Job drawing, mm, ordinate dimensions from the low corner. One solid piece. Give positions to 0.01 mm unless a question says otherwise; leave off trailing zeros. Write each loop counter-clockwise with the first axis right and the second up, starting at its lowest first coordinate (ties: lowest second). Pieces come first, ordered by that corner, then holes. Notation, with made-up numbers: (-6.5, -19) - (0.5, -19) arc R25 ccw to (0.5, 14) - close; hole circle Ø8 at (14.25, -17). An arc over 180 degrees is marked (long way). Answer as a JSON object with one key per item and string values.
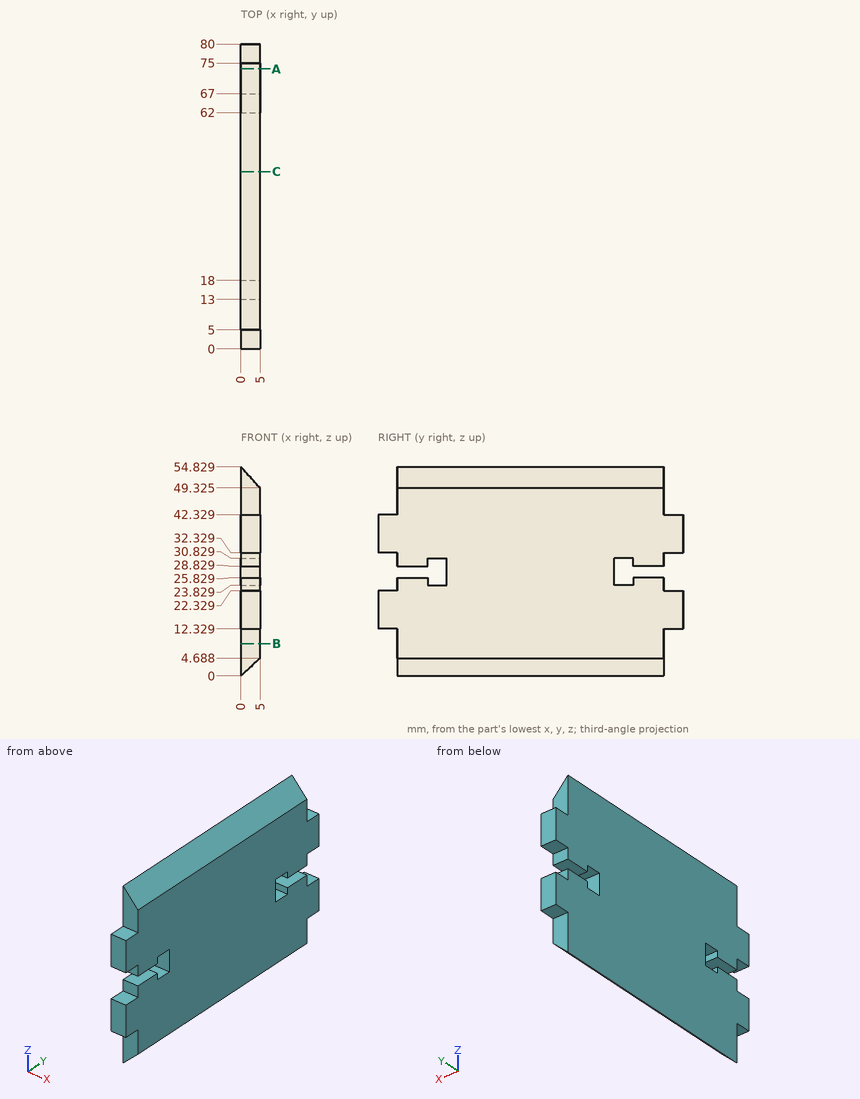
Item 1: Cut at C-C (y = 46.5). Give the cut face in (x, z) (3 decimals), and give its area (3 significant figures).
Entries:
{"outline": "(0, 0) - (5, 4.688) - (5, 49.325) - (0, 54.829) - close", "area": "249 mm2"}
Item 2: Flat gauge pins, fed straight in: P1, Ø1.5, axis at x = 3.5, z = 4.5, coming from the -Y side; P2, Ø2.5, axis at x = 3, y = 63.5, coming from the +Z side; P3, Ø1.5, axis at x = 3.5, y = 70.5, coming from the +Z side. Where does each tip first touch, or does it go through?
Entries:
{"P1": "y = 5", "P2": "z = 52.9", "P3": "z = 51.8"}
Item 3: Cut at B-B (z = 8.5). Give the cut face in (x, y).
Entries:
{"outline": "(0, 5) - (5, 5) - (5, 75) - (0, 75) - close"}
Item 4: Probe line 1 (Y direction, x = 1.9, z = 24.5); line 2 (Y direction, x = 4.25, z = 22.5); line 3 (Z direction, x = 2.95, y = 17.5). List the from-to ranges inside material, lowest first. Write a range as from..to.
Entries:
{"line 1": "5..13, 18..62, 67..75", "line 2": "5..75", "line 3": "2.77..23.83, 30.83..51.58"}
Item 5: Cut at A-A (y = 73.5). Give the cut face in (x, z) (3 decimals), and give its area (3 significant figures).
Entries:
{"outline": "(0, 0) - (5, 4.688) - (5, 25.829) - (0, 25.829) - close; (0, 28.829) - (5, 28.829) - (5, 49.325) - (0, 54.829) - close", "area": "234 mm2"}
